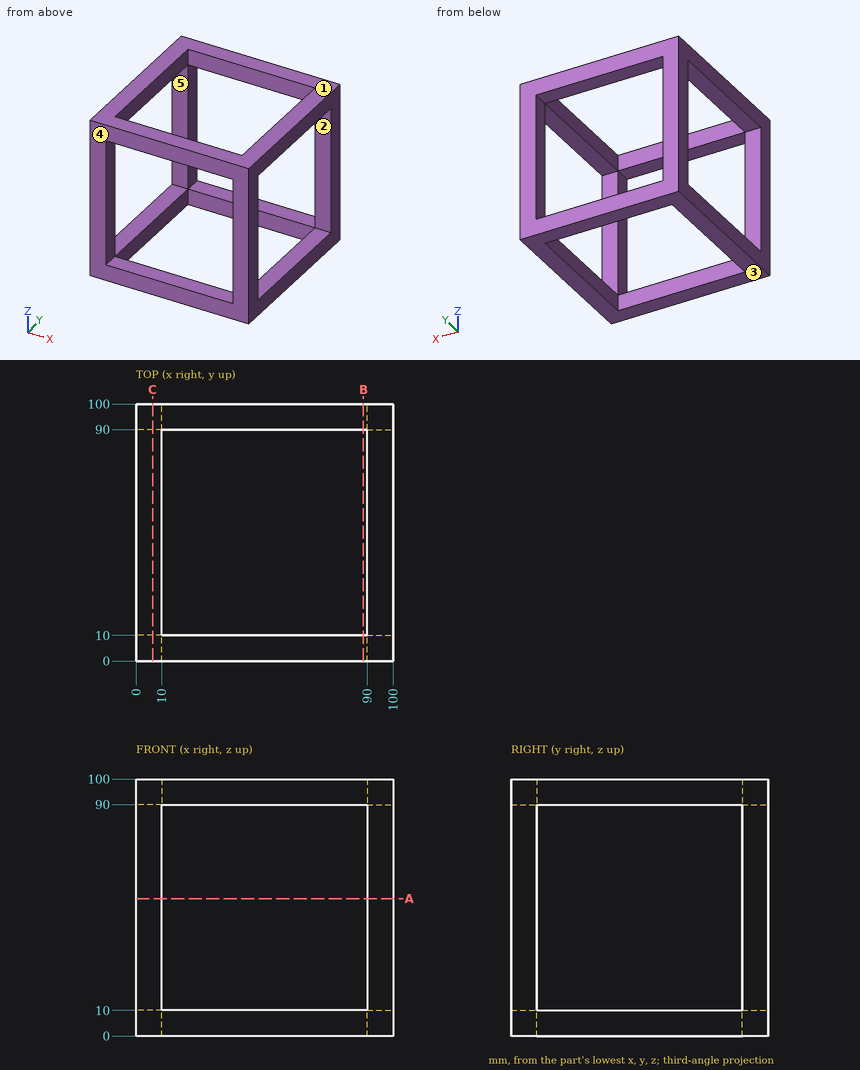
Geometry check sheet. Reference: drawing and pictorial views, mm from the part's lowest x, y, z. A direction names the side the tool comes from. Round coordinates to 2 decimals unless told otherwise and drop trailing zeros. Loops run counter-clockwise (first coordinate to the right, second up) from the corner with the lowest first, then second, coordinate; pieces in that order, holes last. Notation, with made-up numbers: M 25.5,-11 L 74.5,-11 A13 cw 74.5,8 Z; hole C 72,31 d9. An arc over 180 degrees is marked long. Return JSON: item names as keys, results as strings. Group by question number.
(1) Go/stop test with a flat-tipped pin: pin 1 (3 mm diameter, centred on y = 47.5, z = 95.5, fed in from -X). Record where the tip stops, or that it passes through.
(2) Mould release check, pull along Z, two halves, no side actions. Record for the marked faces 3, 4 and 5: pulls with the +Z half, pulls with the -Z half, needs draft (parallel to the pull), parting line crosses it, or undercut.
(3) Scan line: line 1 along Z through (x, y) = (50.5, 7). Record every from-to range of solid material in increasing order. Write a range as [from, to].
(4) Set-up check for the marked faces 1 and 2: record each of +Z, -Z, +X, -X, +Y, -Y from which the full face is reachable in a straight line by a thin tool's end or side.
(5) Section check A-A, the plane z = 53.5. Enter the section's corners in (x, y), and give its area (3 significant figures).
(6) Section check C-C, the plane x = 6.5. Enter the section's corners in (y, z), and give its area (3 significant figures).
Data:
{
 "1": {"pin 1": "x = 0"},
 "2": {"face 3": "pulls with the -Z half", "face 4": "needs draft", "face 5": "undercut"},
 "3": {"line 1": "[0, 10], [90, 100]"},
 "4": {"face 1": "+Z, +X, -X, +Y, -Y", "face 2": "+X, -X"},
 "5": {"outline": "M 0,0 L 10,0 L 10,10 L 0,10 Z; M 0,90 L 10,90 L 10,100 L 0,100 Z; M 90,0 L 100,0 L 100,10 L 90,10 Z; M 90,90 L 100,90 L 100,100 L 90,100 Z", "area": "400 mm²"},
 "6": {"outline": "M 0,0 L 100,0 L 100,100 L 0,100 Z; hole M 10,10 L 90,10 L 90,90 L 10,90 Z", "area": "3,600 mm²"}
}
